Work out the finished part from the listing and answer in its coordinate system (mm). Face numbers are marked on the shaded views. A direction names the side the tool comes from. Round coordinates to 2 decimals unless told otherwise and drop trailing zeros. Loops run counter-clockwise (first coordinate to the right, second up) from the corner with the lowest first, then second, coordinate; pieces in that order, holes last. Notation, with made-up numbers: (2.5, -31) - (35.5, -31) arc R21 ccw to (35.5, -9) - close; hole circle Ø9 at (-24.5, -36). An arc over 180 degrees is marked (long way). Return JSON: item names as keys, results as strings.
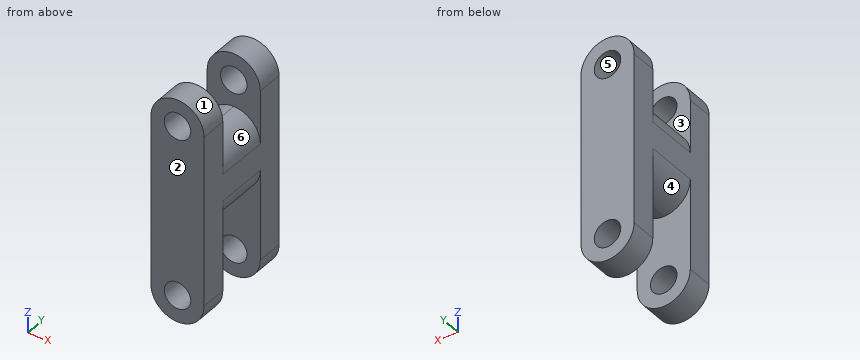
from build123d import *

# Parameters (mm, degrees)
SKETCH1_R           = 2.5
BOSS_EXTRUDE1_DEPTH = 20
SKETCH2_W           = 10
SKETCH2_H           = 10
CUT_EXTRUDE1_DEPTH  = 15
FILLET1_R           = 5
SKETCH3_W           = 25
SKETCH3_H           = 10
CUT_EXTRUDE3_DEPTH  = 10
FILLET3_R           = 5


with BuildPart() as part:
    # Sketch1 → Boss-Extrude1 (new body)
    with BuildSketch(Plane(origin=(0, 0, 0), x_dir=(1, 0, 0), z_dir=(0, 1, 0))):
        with BuildLine():
            Line((-5, 0), (-5, 32))
            ThreePointArc((-5, 32), (0, 37), (5, 32))
            Line((5, 32), (5, 0))
            ThreePointArc((5, 0), (0, -5), (-5, 0))
        make_face()
        with Locations(Location((0, 32, 0), (0, 0, 270))):
            Circle(SKETCH1_R, mode=Mode.SUBTRACT)
        with Locations(Location((0, 0, 0), (0, 0, 270))):
            Circle(SKETCH1_R, mode=Mode.SUBTRACT)
    extrude(amount=BOSS_EXTRUDE1_DEPTH)

    # Sketch2 → Cut-Extrude1 (cut)
    with BuildSketch(Plane(origin=(5, 0, 0), x_dir=(0, 0, -1), z_dir=(1, 0, 0))):
        with Locations((0, 10)):
            Rectangle(SKETCH2_W, SKETCH2_H)
    cut_extrude1 = extrude(amount=-CUT_EXTRUDE1_DEPTH, mode=Mode.SUBTRACT)

    # Mirror1: Cut-Extrude1 across plane
    add(cut_extrude1.mirror(Plane.XY.offset(-15)), mode=Mode.SUBTRACT)

    # Fillet1
    fillet1_edges = [part.edges().sort_by_distance(p)[0] for p in [
        (-5, 10, -25),
        (5, 10, -25),
        (-5, 10, -5),
        (5, 10, -5),
    ]]
    fillet(fillet1_edges, radius=FILLET1_R - 0.0001)  # a hair under: the kernel refuses the full size

    # Sketch3 → Cut-Extrude3 (cut)
    with BuildSketch(Plane(origin=(5, 0, 0), x_dir=(0, 0, -1), z_dir=(1, 0, 0))):
        with Locations((32.5, 10)):
            Rectangle(SKETCH3_W, SKETCH3_H)
    extrude(amount=-CUT_EXTRUDE3_DEPTH, mode=Mode.SUBTRACT)

    # Fillet3
    fillet3_edges = [part.edges().sort_by_distance(p)[0] for p in [
        (-5, 10, -20.0001),
        (5, 10, -20.0001),
    ]]
    fillet(fillet3_edges, radius=FILLET3_R - 0.0001)  # a hair under: the kernel refuses the full size


solid = part.part
1) Find the intervals of material crossed by L1, parallel to Z at x = 0, y = 2.65; L2, parallel to Y at x = -1.75, z = -26; L3, parallel to X at y = 17.75, z = -32, in increasing order.
Verdict:
{"L1": "z = -37 to -34.5, -29.5 to -2.5, 2.5 to 5", "L2": "y = 0 to 5, 15 to 20", "L3": "x = -5 to -2.5, 2.5 to 5"}
2) Section C-C (z = -28) is taken. Give the vertices of the cut face in (x, y), and give its area (3 significant figures).
Verdict:
{"outline": "(-5, 0) - (5, 0) - (5, 5) - (-5, 5) - close; (-5, 15) - (5, 15) - (5, 20) - (-5, 20) - close", "area": "100 mm2"}
3) Section D-D (x = -1.75) is taken. Give the vertices of the cut face in (y, z), and give its area (3 significant figures).
Verdict:
{"outline": "(0, -36.68) - (5, -36.68) - (5, -33.79) - (0, -33.79) - close; (0, -30.21) - (5, -30.21) - (5, -19.68) - (15, -19.68) - (15, -30.21) - (20, -30.21) - (20, -1.79) - (15, -1.79) - (15, -5.32) - (5, -5.32) - (5, -1.79) - (0, -1.79) - close; (0, 1.79) - (5, 1.79) - (5, 4.68) - (0, 4.68) - close; (15, -36.68) - (20, -36.68) - (20, -33.79) - (15, -33.79) - close; (15, 1.79) - (20, 1.79) - (20, 4.68) - (15, 4.68) - close", "area": "486 mm2"}
4) Determine the mould class of the marked faces 1, 2, 3 and 4 for opening direction Y: pulls with the +Y half, pulls with the -Y half, needs draft (parallel to the pull), parting line crosses it, or undercut.
Verdict:
{"face 1": "needs draft", "face 2": "pulls with the -Y half", "face 3": "undercut", "face 4": "undercut"}
5) A tool of negligible diameter and unlimited length cuts with its end or side. For the marked faces 5 and 6, from which of +Z, -Z, +X, -X, +Y, -Y can it reach the whole face along a straight path? Write none if from no direction.
Verdict:
{"face 5": "+Y, -Y", "face 6": "+Z, +X"}
6) Section B-B (y = 4.5) is taken. Give the vertices of the cut face in (x, z), and give its area (3 significant figures).
Verdict:
{"outline": "(-5, -32) arc R5 ccw to (5, -32) - (5, 0) arc R5 ccw to (-5, 0) - close; hole circle Ø5 at (0, -32); hole circle Ø5 at (0, 0)", "area": "359 mm2"}
7) Flat-ended cylindrical pins translate along their axes: pin 1 (6 mm diameter, centred on y = 13.5, z = -15.5, fed in from +X); pin 2 (1 mm diameter, centred on x = -3, y = 6, fed in from -Z); pin 3 (3 mm diameter, centred on x = -2.5, y = 4.5, fed in from +Z); pin 4 (5 mm diameter, centred on x = -3.5, y = 6, fed in from +Z). Find the tip coordinate at first contact, or state that the pin passes through.
Verdict:
{"pin 1": "stops at x = 5", "pin 2": "stops at z = -19.33", "pin 3": "stops at z = 4.9", "pin 4": "stops at z = 4.85"}
8) Section A-A (z = -2) is taken. Give the vertices of the cut face in (x, y).
Verdict:
{"outline": "(-5, 0) - (-1.5, 0) - (-1.5, 5) - (-5, 5) - close; (-5, 15) - (-1.5, 15) - (-1.5, 20) - (-5, 20) - close; (1.5, 0) - (5, 0) - (5, 5) - (1.5, 5) - close; (1.5, 15) - (5, 15) - (5, 20) - (1.5, 20) - close"}
